Autodesk Inventor part; units mm, degrees
ref_plane "YZ Plane" through (0, 0, 0) normal (1, 0, 0) x (0, 1, 0)
ref_plane "XZ Plane" through (0, 0, 0) normal (0, 1, 0) x (-1, 0, 0)
ref_plane "XY Plane" through (0, 0, 0) normal (0, 0, 1) x (1, 0, 0)
sketch "Sketch1" plane through (0, 0, 0) normal (0, 0, 1) x (1, 0, 0)
  circle A0 centre (0, 0) radius 15
  circle A1 centre (0, 0) radius 23
  dimension "d0" = 30
  dimension "d1" = 46
extrude "Extrusion1" add sketch "Sketch1" along normal blind 1
sketch "Sketch2" plane through (0, 0, 1) normal (0, 0, 1) x (1, 0, 0)
  line L0 (0, 0) -> (23, 0) construction
  circle A0 centre (0, 0) radius 23
  circle A1 centre (0, 0) radius 20.5 construction
  line L1 (0, 0) -> (14.4957, 14.4957) construction
  dimension "d35" = 41
  dimension "d34" = 45
hole "For-m3-screws" at (14.4957, 14.4957, 1) direction (0, 0, -1) diameter 3.2 end through all
pattern_circular "Circular Pattern1" count 4 over 360 about axis through (0, 0, 0) along (0, 0, 1) of "For-m3-screws"
sketch "Sketch4" plane through (0, 0, 0) normal (0, 0, 1) x (1, 0, 0)
  line L0 (21, 30) -> (26, 30)
  line L1 (26, 30) -> (26, -30)
  line L2 (26, -30) -> (21, -30)
  line L3 (21, -30) -> (21, 30)
  point P0 (0, 0)
  point P1 (26, 0)
  dimension "d19" = 21
  dimension "d20" = 60
  dimension "d21" = 5
extrude "Extrusion3" cut sketch "Sketch4" along normal blind 10
mirror "Mirror1" about plane through (0, 0, 0) normal (1, 0, 0) of "Extrusion3"
equation "\"d0\" = innerdiameter"
equation "\"d1\" = outerdiameter"
equation "\"d35\" = holepositiondiameter"
equation "\"outerdiameter\" = 46"
equation "\"innerdiameter\" = 30"
equation "\"holepositiondiameter\" = 41"
equation "\"trimspan\" = 21"
properties part number "boron window" material "Stainless Steel"
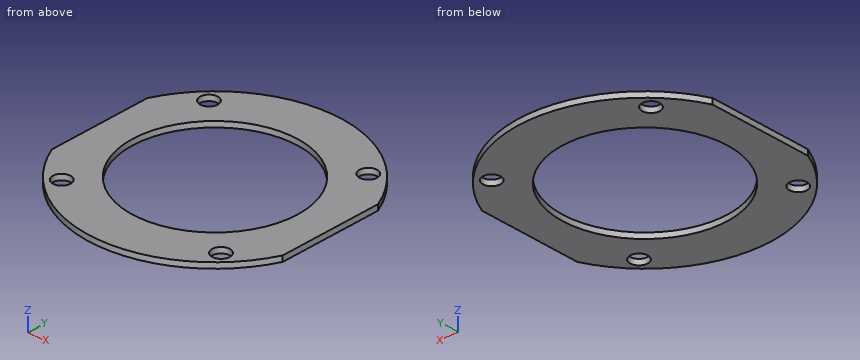
Here's how the part is built. I have some questions about the finished solid (model axes, mm). Coordinates: 2 decimals unless noted, no trailing zeros. Order: outer loops, then holes, each group sorted by start corner. A loop starts at its lowest first (then second) coordinate and runs counter-clockwise, first axis right, second up. Notation, with made-up numbers: (40, 74) -> (53, 74) arc R27 cw to (53, 92) -> close; hole circle Ø7 at (27.25, 34). An arc over 180 degrees is marked (long way). Return JSON: item names as keys, results as strings.
1) If we section it at C-C on z = 0.55: List the corners of the cut face in (x, y) for me, plus the area to 3 significant figures.
Conclusion:
{"outline": "(-21, -9.38) arc R23 ccw to (21, -9.38) -> (21, 9.38) arc R23 ccw to (-21, 9.38) -> close; hole circle Ø3.2 at (-14.5, -14.5); hole circle Ø3.2 at (-14.5, 14.5); hole circle Ø30 at (0, 0); hole circle Ø3.2 at (14.5, -14.5); hole circle Ø3.2 at (14.5, 14.5)", "area": "872 mm²"}
2) If we section it at B-B on y = 0: List the corners of the cut face in (x, z) for me.
Conclusion:
{"outline": "(-21, 0) -> (-15, 0) -> (-15, 1) -> (-21, 1) -> close; (15, 0) -> (21, 0) -> (21, 1) -> (15, 1) -> close"}
3) If we section it at A-A on x = -9.5: List the corners of the cut face in (y, z) for me.
Conclusion:
{"outline": "(-20.95, 0) -> (-11.61, 0) -> (-11.61, 1) -> (-20.95, 1) -> close; (11.61, 0) -> (20.95, 0) -> (20.95, 1) -> (11.61, 1) -> close"}
4) If we section it at D-D on y = -18: List the corners of the cut face in (x, z) for me.
Conclusion:
{"outline": "(-14.32, 0) -> (14.32, 0) -> (14.32, 1) -> (-14.32, 1) -> close"}
5) If I drill on probe 1 along Y at (x, z) = (0, 0.8); probe 2 along X at (y, z) = (-2, 0.8); probe 3 along Y at (x, z) = (-7, 0.1), over which ranges is the centre line in solid material (lowest first)?
Conclusion:
{"probe 1": "y = -23 to -15, 15 to 23", "probe 2": "x = -21 to -14.87, 14.87 to 21", "probe 3": "y = -21.91 to -13.27, 13.27 to 21.91"}
